Could you check a few things on this drawing? It's one solid part, dimensions in mm from its lowest x, y, z. A direction names the side the tool comes from. Give positions to 0.01 mm unless a question says otherwise; leave off trailing zeros. Order: outer loops, then holes, each group sorted by start corner. A loop starts at its lowest first (then second) coordinate and runs counter-clockwise, first axis right, second up.
(1) On a 3-axis mill with a long thin cutter (end or side, diameter ignored), from which of +Z, -Z, +X, -X, +Y, -Y can I reach the whole of each face in a straight line? I mean the marked faces 1 and 2. Say none if no direction works.
(2) Imagine slicing it at B-B, the plane y = 0.8. Write out the boundary of the cut face in (x, z).
(3) Will these pins go through, and if not, where does the flat tip stop? pin 1 (2 mm diameter, centred on y = 0.5, z = 1.5, fed in from -X); pin 2 (2.5 mm diameter, centred on x = 3.85, z = 3.85, fed in from -Y).
(4) If we mould it in two halves opening along X, with no side actions, what happens to the marked faces 3, 4 and 5? For each: released by +X, released by -X, zero draft, split by the parting line, or undercut.
(5) Imagine slicing it at A-A, the plane z = 3.85. Write out the boundary of the cut face in (x, y), then the cut area to 3 significant figures.
(6) Imagine slicing it at C-C, the plane y = 3. Write out the boundary of the cut face in (x, z).
(7) If I drill on probe 1 along Z at (x, y) = (3.85, 1.8); probe 2 along Z at (x, y) = (3.85, 0.8); probe 3 along Y at (x, z) = (4.25, 3.5), over which ranges is the centre line in solid material (lowest first)?
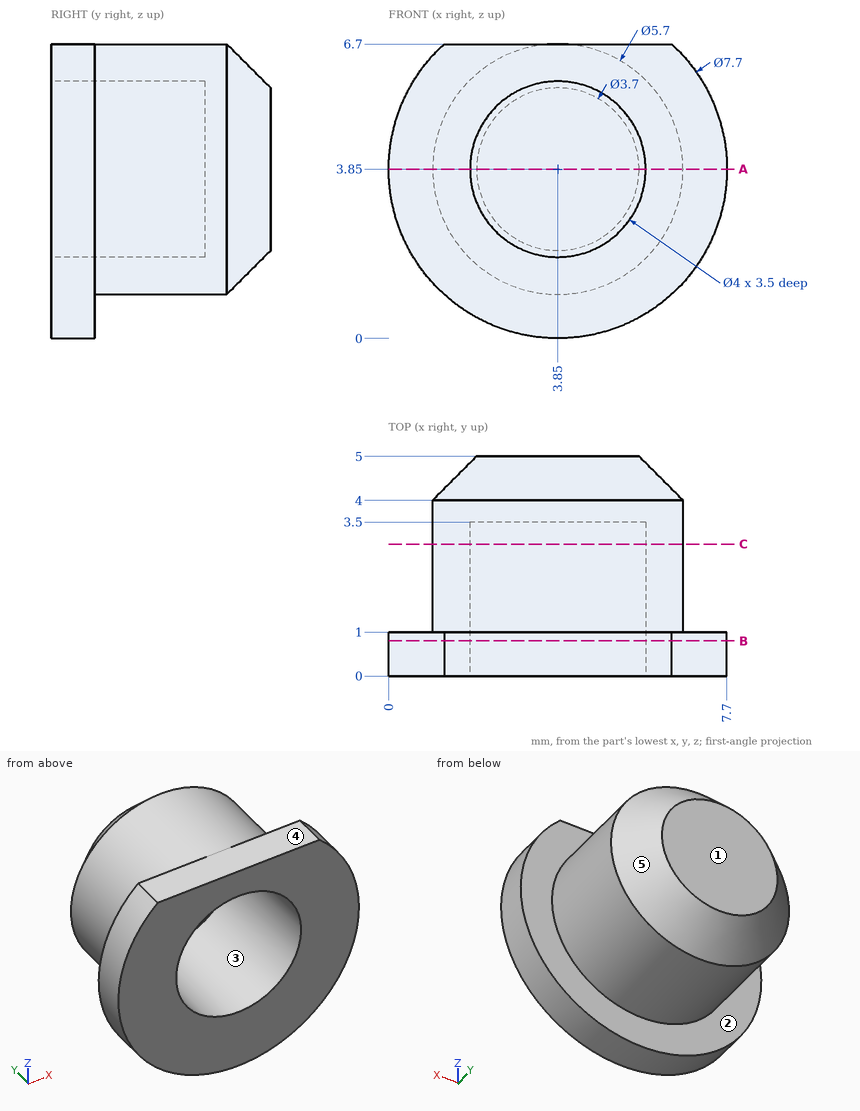
Answer block:
1. face 1: +Z, -Z, +X, -X, +Y
1. face 2: +Y
2. outline: (1.26, 6.7) arc R3.85 ccw (long way) to (6.44, 6.7) - close; hole circle Ø4 at (3.85, 3.85)
3. pin 1: stops at x = 0.24
3. pin 2: stops at y = 3.5
4. face 3: undercut
4. face 4: zero draft
4. face 5: split by the parting line
5. outline: (0, 0) - (1.85, 0) - (1.85, 3.5) - (5.85, 3.5) - (5.85, 0) - (7.7, 0) - (7.7, 1) - (6.7, 1) - (6.7, 4) - (5.7, 5) - (2, 5) - (1, 4) - (1, 1) - (0, 1) - close
5. area: 15.5 mm2
6. outline: circle Ø5.7 at (3.85, 3.85); hole circle Ø4 at (3.85, 3.85)
7. probe 1: z = 1 to 1.85, 5.85 to 6.7
7. probe 2: z = 0 to 1.85, 5.85 to 6.7
7. probe 3: y = 3.5 to 5
